```python
from build123d import *

# Parameters (mm, degrees)
SKETCH1_R           = 15
BOSS_EXTRUDE1_DEPTH = 130
SKETCH7_R           = 40
SKETCH7_R_2         = 20
BOSS_EXTRUDE2_DEPTH = 15


with BuildPart() as part:
    # Sketch1 → Boss-Extrude1 (new body)
    with BuildSketch(Plane(origin=(0, 0, 0), x_dir=(0, 0, -1), z_dir=(1, 0, 0))):
        Circle(SKETCH1_R)
    extrude(amount=BOSS_EXTRUDE1_DEPTH)

    # Sketch4 → Revolve1 (revolve)
    with BuildSketch(Plane.XY):
        with BuildLine():
            Line((-20, 0), (20, 0))
            ThreePointArc((20, 0), (0, 20), (-20, 0))
        make_face()
    revolve(axis=Axis((0, 0, 0), (1, 0, 0)))

    # Sketch7 → Boss-Extrude2 (add, symmetric)
    with BuildSketch(Plane(origin=(0, 0, 0), x_dir=(1, 0, 0), z_dir=(0, 1, 0))):
        with Locations((167.080992435, 0)):
            Circle(SKETCH7_R)
        with Locations(Location((167.080992435, 0, 0), (0, 0, 270))):
            Circle(SKETCH7_R_2, mode=Mode.SUBTRACT)
    extrude(amount=BOSS_EXTRUDE2_DEPTH, both=True)


solid = part.part
```
Part model, mm, in its own coordinate system. A direction names the side the tool comes from. Round coordinates to 2 decimals unless told otherwise and drop trailing zeros. Order: outer loops, then holes, each group sorted by start corner. A loop starts at its lowest first (then second) coordinate and runs counter-clockwise, first axis right, second up. Notation, with made-up numbers: M 8.25,-21.75 L 52.25,-21.75 A31 ccw 52.25,15.25 Z; hole C -22.75,79 d6. An arc over 180 degrees is marked long. Answer in a Markdown table with one row per item. Add a question column.
Q1. Pin check, flat tips, straight feed: pin 1 (1.5 mm diameter, centred on x = 123, z = -5, fed in from -Y); pin 2 (5 mm diameter, centred on y = -13.5, z = -30.5, fed in from +X); pin 3 (10 mm diameter, centred on x = 32, z = 4, fed in from -Y). Stop position of each tip, or through.
Q2. Cut at D-D on z = -30.5. Give the cut face in (x, y), and give its area (3 significant figures).
Q3. 3-axis set-ups, long thin cutter, end or side, ignore diameter. For faces 1 (the face through (148.7, 15, 8.3)), 2 (the face through (154.91, -0.21, -15.87)): which of +Z, -Z, +X, -X, +Y, -Y reach the whole face in a straight line?
Q4. Mould opens along X. For faces 3 (the face through (70.797, 0.66, 14.985)), 4 (the face through (148.7, -15, 8.3)) say: +X half, -X half, draft (parallel to the pull), parting line (faces both ways), or undercut.
Q5. Wall check: L1, parallel to X at y = 1.25, z = 0; L2, parallel to X at y = 8.5, z = -16; L3, parallel to X at y = -7.5, z = 0. Give the ranges that are in metal, low to high. Write a range as from..to.
Q6. Cut at A-A on z = 17. Give the cut face in (x, y).
Q7. Cut at C-C on x = 38.5. Give the cut face in (y, z).
Q8. Cut at B-B on y = 0. Give the cut face in (x, z), and give its area (3 significant figures).
Established:
| question | item | result |
|---|---|---|
| 1 | pin 1 | stops at y = -14.39 |
| 1 | pin 2 | stops at x = 195.65 |
| 1 | pin 3 | stops at y = -15 |
| 2 | outline | M 141.2,-15 L 192.96,-15 L 192.96,15 L 141.2,15 Z |
| 2 | area | 1,550 mm2 |
| 3 | face 1 | +Z, -Z, +X, +Y |
| 3 | face 2 | +Y, -Y |
| 4 | face 3 | undercut |
| 4 | face 4 | draft |
| 5 | L1 | x = -19.96..147.08, 187.08..207.08 |
| 5 | L2 | x = -8.47..8.47, 130.42..155.08, 179.08..203.74 |
| 5 | L3 | x = -18.54..147.08, 187.08..207.08 |
| 6 | outline | C 0,0 d21.07; M 130.87,-15 L 156.55,-15 L 156.55,15 L 130.87,15 Z; M 177.62,-15 L 203.29,-15 L 203.29,15 L 177.62,15 Z |
| 7 | outline | C 0,0 d30 |
| 8 | outline | M 13.23,-15 L 130,-15 A40 ccw long 130,15 L 13.23,15 A20 ccw long Z; hole C 167.08,0 d40 |
| 8 | area | 8,330 mm2 |
